Verification items for the finished model (mm, model axes). A direction names the side the tool comes from. Round coordinates to 2 decimals unless told otherwise and drop trailing zeros. Write each loop counter-clockwise with the first axis right and the second up, starting at its lowest first coordinate (ties: lowest second). Pieces come first, ordered by that corner, then holes. Notation, with made-up numbers: (37, 29.25) - (72, 29.25) arc R19 ccw to (72, 43.25) - close; hole circle Ø10 at (23, 40). An arc over 180 degrees is marked (long way). Answer as a JSON object with one key per item and string values.
```python
from build123d import *
from build123d.topology import SkipClean

# Parameters (mm, degrees)
SKETCH1_W               = 35.56
SKETCH1_H               = 25.4
BOSS_EXTRUDE1_DEPTH     = 25.4
SKETCH2_R               = 6.35
BOSS_EXTRUDE2_DEPTH     = 25.4
SKETCH4_R               = 1.395358984
CUT_EXTRUDE1_DEPTH      = 5.842
SKETCH7_W               = 35.56
SKETCH7_H               = 25.4
BOSS_EXTRUDE3_DEPTH     = 101.6
CUT_EXTRUDE2_DEPTH      = 142.44402285
CUT_EXTRUDE2_DEPTH_BACK = 12.7
SKETCH4_4_R             = 1.395358984
SKETCH10_W              = 25.4
SKETCH10_H              = 50.8
BOSS_EXTRUDE4_DEPTH     = 31.75
SKETCH11_W              = 20.32
SKETCH11_H              = 37.592
CUT_EXTRUDE3_DEPTH      = 49.53


with BuildPart() as part:
    # Sketch1 → Boss-Extrude1 (new, symmetric)
    with BuildSketch(Plane(origin=(0, 0, 0), x_dir=(1, 0, 0), z_dir=(0, 1, 0))):
        Rectangle(SKETCH1_W, SKETCH1_H)
    extrude(amount=BOSS_EXTRUDE1_DEPTH, both=True)

    # Sketch2 → Boss-Extrude2 (add, symmetric)
    with BuildSketch(Plane.ZY.offset(17.78)):
        with Locations(Location((0, 19.05, 0), (0, 0, 90))):
            Circle(SKETCH2_R)
    extrude(amount=BOSS_EXTRUDE2_DEPTH, both=True)

    # Sketch4 → Cut-Extrude1 (cut)
    with BuildSketch(Plane(origin=(17.78, 0, 0), x_dir=(0, 0, -1), z_dir=(1, 0, 0))):
        with BuildLine():
            ThreePointArc((-5.7416, 14.7838), (-4.273649798, 11.982116734), (-3.767, 8.86))
            Line((-3.767, 8.86), (-3.767, -5.29))
            ThreePointArc((-3.767, -5.29), (0.16, -9.217), (4.087, -5.29))
            Line((4.087, -5.29), (4.087, 8.86))
            ThreePointArc((4.087, 8.86), (4.593649798, 11.982116734), (6.0616, 14.7838))
            ThreePointArc((6.0616, 14.7838), (7.15843669, 16.87718777), (7.537, 19.21))
            Line((7.537, 19.21), (7.537, 26.587))
            Line((7.537, 26.587), (-7.217, 26.587))
            Line((-7.217, 26.587), (-7.217, 19.21))
            ThreePointArc((-7.217, 19.21), (-6.83843669, 16.87718777), (-5.7416, 14.7838))
        make_face()
        with Locations((0.16, -5.29)):
            Circle(SKETCH4_R, mode=Mode.SUBTRACT)
        with Locations((0.16, -1.29)):
            Circle(SKETCH4_R, mode=Mode.SUBTRACT)
    extrude(amount=-CUT_EXTRUDE1_DEPTH, mode=Mode.SUBTRACT)

    # Sketch7 → Boss-Extrude3 (add)
    with SkipClean():  # the faces are left unmerged after this step: merging them gives an invalid solid
        with BuildSketch(Plane.XZ.offset(25.4)):
            Rectangle(SKETCH7_W, SKETCH7_H)
        extrude(amount=BOSS_EXTRUDE3_DEPTH)

    # Sketch4_4 → Cut-Extrude2 (cut, two sides: drawn at the far end of the back side and taken through both)
    with SkipClean():  # the faces are left unmerged after this step: merging them gives an invalid solid
        with BuildSketch(Plane(origin=(17.78, 0, 0), x_dir=(0, 0, -1), z_dir=(1, 0, 0)).offset(-CUT_EXTRUDE2_DEPTH_BACK)):
            with Locations(Location((0.16, -1.29, 0), (0, 0, 180))):
                Circle(SKETCH4_4_R)
            with Locations(Location((0.16, -5.29, 0), (0, 0, 180))):
                Circle(SKETCH4_4_R)
        extrude(amount=CUT_EXTRUDE2_DEPTH + CUT_EXTRUDE2_DEPTH_BACK, mode=Mode.SUBTRACT)

    # Sketch10 → Boss-Extrude4 (add)
    with SkipClean():  # the faces are left unmerged after this step: merging them gives an invalid solid
        with BuildSketch(Plane.ZY.offset(17.78)):
            with Locations((0, -101.6)):
                Rectangle(SKETCH10_W, SKETCH10_H)
        extrude(amount=BOSS_EXTRUDE4_DEPTH)

    # Sketch11 → Cut-Extrude3 (cut)
    with SkipClean():  # the faces are left unmerged after this step: merging them gives an invalid solid
        with BuildSketch(Plane(origin=(17.78, 0, 0), x_dir=(0, 0, -1), z_dir=(1, 0, 0))):
            with Locations((0, -105.156)):
                Rectangle(SKETCH11_W, SKETCH11_H)
        extrude(amount=-CUT_EXTRUDE3_DEPTH, mode=Mode.SUBTRACT)


solid = part.part
```
Q1. Section check B-B, the plane y = -106.5. Record the cut outline in (x, z), then the cut area to 3 significant figures.
Geometry check:
{"outline": "(-49.53, -12.7) - (17.78, -12.7) - (17.78, -10.16) - (-31.75, -10.16) - (-31.75, 10.16) - (17.78, 10.16) - (17.78, 12.7) - (-49.53, 12.7) - close", "area": "703 mm2"}
Q2. Section check A-A, the plane x = 9. Record the cut outline in (y, z), then the cut area to 3 significant figures.
Geometry check:
{"outline": "(-127, -12.7) - (25.4, -12.7) - (25.4, 12.7) - (-127, 12.7) - close; hole (-123.95, -10.16) - (-86.36, -10.16) - (-86.36, 10.16) - (-123.95, 10.16) - close; hole circle Ø2.79 at (-5.29, -0.16); hole circle Ø2.79 at (-1.29, -0.16)", "area": "3,090 mm2"}
Q3. Material ranges on line 1 along Y through (x, z) = (8.25, -0.16); line 2 along Y through (x, z) = (6, -6); line 3 along Z through (x, y) = (-9.5, -106), recorded low to high. Write a range as [from, to].
Geometry check:
{"line 1": "y = [-127, -123.95], [-86.36, -6.69], [-3.89, -2.69], [0.11, 25.4]", "line 2": "y = [-127, -123.95], [-86.36, 25.4]", "line 3": "z = [-12.7, -10.16], [10.16, 12.7]"}
Q4. Section check C-C, the plane y = 4.5. Record the cut outline in (x, z).
Geometry check:
{"outline": "(-17.78, -12.7) - (17.78, -12.7) - (17.78, -4.09) - (11.94, -4.09) - (11.94, 3.77) - (17.78, 3.77) - (17.78, 12.7) - (-17.78, 12.7) - close"}
Q5. Gauge pin test, flat ends, axial feed: P1, Ø10, axis at y = -102.5, z = -0.5, coming from the +X side; P2, Ø0.8, axis at y = -2, z = -0.5, coming from the +X side; P3, Ø4.5, axis at y = -5.29, z = -0.16, coming from the +X side. Record the tip position at first contact, or that the pin passes through.
Geometry check:
{"P1": "stops at x = -31.75", "P2": "stops at x = 5.08", "P3": "stops at x = 11.94"}
Q6. Set-up check for faces 5 (the flat face through (-31.75, -105, 0)), 6 (the flat face through (15, 22, 7.217)), 7 (the flat face through (-33, -76.2, 0)): record each of +Z, -Z, +X, -X, +Y, -Y from which the full face is reachable in a straight line by a thin tool's end or side.
Geometry check:
{"face 5": "+X", "face 6": "+X, +Y", "face 7": "+Z, -Z, -X"}
Q7. Release check for a two-part mould opening along Z. For faces 1 (the cylindrical face through (-30.658, 25.107, -1.907)), 2 (the flat face through (-7, -105, 10.16)), 3 (the flat face through (-43.18, 19, 0)), 4 (the cylindrical face through (14.9, 12.024, 4.288)) record: released by +Z, released by -Z, zero draft, split by the parting line, or undercut.
Geometry check:
{"face 1": "split by the parting line", "face 2": "undercut", "face 3": "zero draft", "face 4": "undercut"}
Q8. Section check D-D, the plane y = -66.5. Record the cut outline in (x, z).
Geometry check:
{"outline": "(-17.78, -12.7) - (17.78, -12.7) - (17.78, 12.7) - (-17.78, 12.7) - close"}
